Work out the finished part from the listing and answer in its coordinate system (mm). Coordinates: 2 decimals unless noted, no trailing zeros. Write each loop counter-clockwise with the first axis right and the second up, starting at its lowest first coordinate (ties: lowest second). Pieces come first, ordered by that corner, then holes. Notation, with made-up numbers: M 15,-26 L 54,-26 A11 cw 54,-12 Z; hole C -27.5,48 d2. An arc over 180 degrees is marked long. Answer as CSV lines item,"result". Start each with the question number.
(1) The mould has two halves that part along Z. Classify faces 1 (the cylindrical face through (-13, 1, -7)), 2 (the flat face through (-1, 0, -3)), 3 (the flat face through (36, 1, 29)): released by +Z, released by -Z, zero draft, split by the parting line, or undercut.
(2) A cutting plane is placed at A-A on x = -15. Give the vertices of the cut face in (y, z).
(3) A cutting plane is placed at D-D on y = 1.45. Count the separate pieces of the cut face and the enclosed holes in it, then the cut area to 3 significant figures.
(4) Find the intervals of material crossed by L1, parallel to Z at x = 10, y = 0.1; L2, parallel to Z at x = 14, y = 0.75; L3, parallel to Z at x = 47, y = 0.85, in increasing order. Write a range as [from, to].
(5) A cutting plane is placed at C-C on z = 25. Give the vertices of the cut face in (x, y), then the cut area to 3 significant figures.
(6) A cutting plane is placed at B-B on x = -46. Give the vertices of the cut face in (y, z).
(7) A flat-ended cylindrical pin translates along its axis: P1, Ø10, axis at x = 13.5, z = 6, coming from the -Y side. Find the tip coordinate at first contact, or state that the pin passes through.
from build123d import *

# Parameters (mm, degrees)
SKETCH_1_R      = 1.5
SKETCH_1_R_2    = 0.925
SKETCH_1_R_3    = 1
SKETCH_1_R_4    = 15
SKETCH_1_R_5    = 2.5
SKETCH_1_R_6    = 6.425
EXTRUDE_1_DEPTH = 2
FILLET_1_R      = 0.75


with BuildPart() as part:
    # 草图1 → 凸台-拉伸1 (new body)
    # profile 1 of 11: a face of its own
    with BuildSketch(Plane(origin=(0, 0, 0), x_dir=(1, 0, 0), z_dir=(0, 1, 0))):
        Polygon((-19.848034865, 26.695013128), (-30, 23), (30, 23), (19.848034865, 26.695013128), (0.026493373, 26.695013128), (-0.026493373, 26.695013128), align=None)
    # profile 2 of 11: a face of its own
    with BuildSketch(Plane(origin=(0, 0, 0), x_dir=(1, 0, 0), z_dir=(0, 1, 0))):
        Polygon((-19.848034865, 26.695013128), (-30, 23), (30, 23), (19.848034865, 26.695013128), (0.026493373, 26.695013128), (-0.026493373, 26.695013128), align=None)
    # profile 3 of 11: a face of its own
    with BuildSketch(Plane(origin=(0, 0, 0), x_dir=(1, 0, 0), z_dir=(0, 1, 0))):
        Polygon((-30, 23), (-50, 23), (-50, 7), (-50, -1), (-50, -5), (-50, -23), (-42, -23), (42, -23), (50, -23), (50, -5), (50, -1), (50, 7), (50, 23), (30, 23), align=None)
        with Locations(Location((-46, -15, 0), (0, 0, 270))):
            Circle(SKETCH_1_R, mode=Mode.SUBTRACT)
        with Locations(Location((-42, -15, 0), (0, 0, 270))):
            Circle(SKETCH_1_R_2, mode=Mode.SUBTRACT)
        with Locations(Location((-30.7465, -13.935, 0), (0, 0, 270))):
            Circle(SKETCH_1_R, mode=Mode.SUBTRACT)
        with Locations(Location((-12.727922061, -5.727922061, 0), (0, 0, 270))):
            Circle(SKETCH_1_R_3, mode=Mode.SUBTRACT)
        with BuildLine():
            ThreePointArc((-20.969611628, -19), (-22.969611628, -17), (-20.969611628, -15))
            Line((-20.969611628, -15), (20.969611628, -15))
            ThreePointArc((20.969611628, -15), (22.969611628, -17), (20.969611628, -19))
            Line((20.969611628, -19), (-20.969611628, -19))
        make_face(mode=Mode.SUBTRACT)
        with Locations(Location((30.7465, -13.935, 0), (0, 0, 270))):
            Circle(SKETCH_1_R, mode=Mode.SUBTRACT)
        with BuildLine():
            ThreePointArc((-6, -13), (-7.5, -11.5), (-6, -10))
            Line((-6, -10), (6, -10))
            ThreePointArc((6, -10), (7.5, -11.5), (6, -13))
            Line((6, -13), (-6, -13))
        make_face(mode=Mode.SUBTRACT)
        with Locations(Location((12.727922061, -5.727922061, 0), (0, 0, 270))):
            Circle(SKETCH_1_R_3, mode=Mode.SUBTRACT)
        with Locations(Location((42, -15, 0), (0, 0, 270))):
            Circle(SKETCH_1_R_2, mode=Mode.SUBTRACT)
        with Locations(Location((46, -15, 0), (0, 0, 270))):
            Circle(SKETCH_1_R, mode=Mode.SUBTRACT)
        with Locations(Location((-46, 0, 0), (0, 0, 270))):
            Circle(SKETCH_1_R, mode=Mode.SUBTRACT)
        with Locations(Location((-42, 0, 0), (0, 0, 270))):
            Circle(SKETCH_1_R_2, mode=Mode.SUBTRACT)
        with Locations(Location((-46, 15, 0), (0, 0, 270))):
            Circle(SKETCH_1_R, mode=Mode.SUBTRACT)
        with Locations(Location((-42, 15, 0), (0, 0, 270))):
            Circle(SKETCH_1_R_2, mode=Mode.SUBTRACT)
        with Locations(Location((-30.7465, 13.935, 0), (0, 0, 270))):
            Circle(SKETCH_1_R, mode=Mode.SUBTRACT)
        with Locations(Location((-12.727922061, 19.727922061, 0), (0, 0, 270))):
            Circle(SKETCH_1_R_3, mode=Mode.SUBTRACT)
        with Locations((0, 7)):
            Circle(SKETCH_1_R_4, mode=Mode.SUBTRACT)
        with Locations(Location((42, 0, 0), (0, 0, 270))):
            Circle(SKETCH_1_R_2, mode=Mode.SUBTRACT)
        with Locations(Location((46, 0, 0), (0, 0, 270))):
            Circle(SKETCH_1_R, mode=Mode.SUBTRACT)
        with Locations(Location((30.7465, 13.935, 0), (0, 0, 270))):
            Circle(SKETCH_1_R, mode=Mode.SUBTRACT)
        with Locations(Location((12.727922061, 19.727922061, 0), (0, 0, 270))):
            Circle(SKETCH_1_R_3, mode=Mode.SUBTRACT)
        with Locations(Location((42, 15, 0), (0, 0, 270))):
            Circle(SKETCH_1_R_2, mode=Mode.SUBTRACT)
        with Locations(Location((46, 15, 0), (0, 0, 270))):
            Circle(SKETCH_1_R, mode=Mode.SUBTRACT)
    # profile 4 of 11: a face of its own
    with BuildSketch(Plane(origin=(0, 0, 0), x_dir=(1, 0, 0), z_dir=(0, 1, 0))):
        Polygon((-30, 23), (-50, 23), (-50, 7), (-50, -1), (-50, -5), (-50, -23), (-42, -23), (42, -23), (50, -23), (50, -5), (50, -1), (50, 7), (50, 23), (30, 23), align=None)
        with Locations(Location((-46, -15, 0), (0, 0, 270))):
            Circle(SKETCH_1_R, mode=Mode.SUBTRACT)
        with Locations(Location((-42, -15, 0), (0, 0, 270))):
            Circle(SKETCH_1_R_2, mode=Mode.SUBTRACT)
        with Locations(Location((-30.7465, -13.935, 0), (0, 0, 270))):
            Circle(SKETCH_1_R, mode=Mode.SUBTRACT)
        with Locations(Location((-12.727922061, -5.727922061, 0), (0, 0, 270))):
            Circle(SKETCH_1_R_3, mode=Mode.SUBTRACT)
        with BuildLine():
            ThreePointArc((-20.969611628, -19), (-22.969611628, -17), (-20.969611628, -15))
            Line((-20.969611628, -15), (20.969611628, -15))
            ThreePointArc((20.969611628, -15), (22.969611628, -17), (20.969611628, -19))
            Line((20.969611628, -19), (-20.969611628, -19))
        make_face(mode=Mode.SUBTRACT)
        with Locations(Location((30.7465, -13.935, 0), (0, 0, 270))):
            Circle(SKETCH_1_R, mode=Mode.SUBTRACT)
        with BuildLine():
            ThreePointArc((-6, -13), (-7.5, -11.5), (-6, -10))
            Line((-6, -10), (6, -10))
            ThreePointArc((6, -10), (7.5, -11.5), (6, -13))
            Line((6, -13), (-6, -13))
        make_face(mode=Mode.SUBTRACT)
        with Locations(Location((12.727922061, -5.727922061, 0), (0, 0, 270))):
            Circle(SKETCH_1_R_3, mode=Mode.SUBTRACT)
        with Locations(Location((42, -15, 0), (0, 0, 270))):
            Circle(SKETCH_1_R_2, mode=Mode.SUBTRACT)
        with Locations(Location((46, -15, 0), (0, 0, 270))):
            Circle(SKETCH_1_R, mode=Mode.SUBTRACT)
        with Locations(Location((-46, 0, 0), (0, 0, 270))):
            Circle(SKETCH_1_R, mode=Mode.SUBTRACT)
        with Locations(Location((-42, 0, 0), (0, 0, 270))):
            Circle(SKETCH_1_R_2, mode=Mode.SUBTRACT)
        with Locations(Location((-46, 15, 0), (0, 0, 270))):
            Circle(SKETCH_1_R, mode=Mode.SUBTRACT)
        with Locations(Location((-42, 15, 0), (0, 0, 270))):
            Circle(SKETCH_1_R_2, mode=Mode.SUBTRACT)
        with Locations(Location((-30.7465, 13.935, 0), (0, 0, 270))):
            Circle(SKETCH_1_R, mode=Mode.SUBTRACT)
        with Locations(Location((-12.727922061, 19.727922061, 0), (0, 0, 270))):
            Circle(SKETCH_1_R_3, mode=Mode.SUBTRACT)
        with Locations((0, 7)):
            Circle(SKETCH_1_R_4, mode=Mode.SUBTRACT)
        with Locations(Location((42, 0, 0), (0, 0, 270))):
            Circle(SKETCH_1_R_2, mode=Mode.SUBTRACT)
        with Locations(Location((46, 0, 0), (0, 0, 270))):
            Circle(SKETCH_1_R, mode=Mode.SUBTRACT)
        with Locations(Location((30.7465, 13.935, 0), (0, 0, 270))):
            Circle(SKETCH_1_R, mode=Mode.SUBTRACT)
        with Locations(Location((12.727922061, 19.727922061, 0), (0, 0, 270))):
            Circle(SKETCH_1_R_3, mode=Mode.SUBTRACT)
        with Locations(Location((42, 15, 0), (0, 0, 270))):
            Circle(SKETCH_1_R_2, mode=Mode.SUBTRACT)
        with Locations(Location((46, 15, 0), (0, 0, 270))):
            Circle(SKETCH_1_R, mode=Mode.SUBTRACT)
    # profile 5 of 11: a face of its own
    with BuildSketch(Plane(origin=(0, 0, 0), x_dir=(1, 0, 0), z_dir=(0, 1, 0))):
        with Locations((0, 7)):
            Circle(SKETCH_1_R_4)
        with BuildLine():
            ThreePointArc((13, 7), (12.434860091, 3.208660592), (10.788576229, -0.253042323))
            ThreePointArc((10.788576229, -0.253042323), (9.192388155, -2.192388155), (7.253042323, -3.788576229))
            ThreePointArc((7.253042323, -3.788576229), (0, -6), (-7.253042323, -3.788576229))
            ThreePointArc((-7.253042323, -3.788576229), (-9.192388155, -2.192388155), (-10.788576229, -0.253042323))
            ThreePointArc((-10.788576229, -0.253042323), (-13, 7), (-10.788576229, 14.253042323))
            ThreePointArc((-10.788576229, 14.253042323), (-9.192388155, 16.192388155), (-7.253042323, 17.788576229))
            ThreePointArc((-7.253042323, 17.788576229), (0, 20), (7.253042323, 17.788576229))
            ThreePointArc((7.253042323, 17.788576229), (9.192388155, 16.192388155), (10.788576229, 14.253042323))
            ThreePointArc((10.788576229, 14.253042323), (12.434860091, 10.791339408), (13, 7))
        make_face(mode=Mode.SUBTRACT)
    # profile 6 of 11: a face of its own
    with BuildSketch(Plane(origin=(0, 0, 0), x_dir=(1, 0, 0), z_dir=(0, 1, 0))):
        with BuildLine():
            ThreePointArc((7.253042323, -3.788576229), (9.192388155, -2.192388155), (10.788576229, -0.253042323))
            Line((10.788576229, -0.253042323), (4.242640687, 6.292893219))
            ThreePointArc((4.242640687, 6.292893219), (3.949747468, 7), (4.242640687, 7.707106781))
            Line((4.242640687, 7.707106781), (10.788576229, 14.253042323))
            ThreePointArc((10.788576229, 14.253042323), (9.192388155, 16.192388155), (7.253042323, 17.788576229))
            Line((7.253042323, 17.788576229), (0.707106781, 11.242640687))
            ThreePointArc((0.707106781, 11.242640687), (0, 10.949747468), (-0.707106781, 11.242640687))
            Line((-0.707106781, 11.242640687), (-7.253042323, 17.788576229))
            ThreePointArc((-7.253042323, 17.788576229), (-9.192388155, 16.192388155), (-10.788576229, 14.253042323))
            Line((-10.788576229, 14.253042323), (-4.242640687, 7.707106781))
            ThreePointArc((-4.242640687, 7.707106781), (-3.949747468, 7), (-4.242640687, 6.292893219))
            Line((-4.242640687, 6.292893219), (-10.788576229, -0.253042323))
            ThreePointArc((-10.788576229, -0.253042323), (-9.192388155, -2.192388155), (-7.253042323, -3.788576229))
            Line((-7.253042323, -3.788576229), (-0.707106781, 2.757359313))
            ThreePointArc((-0.707106781, 2.757359313), (0, 3.050252532), (0.707106781, 2.757359313))
            Line((0.707106781, 2.757359313), (7.253042323, -3.788576229))
        make_face()
        with Locations(Location((-3.181980515, 3.818019485, 0), (0, 0, 270))):
            Circle(SKETCH_1_R_3, mode=Mode.SUBTRACT)
        with Locations(Location((-3.181980515, 10.181980515, 0), (0, 0, 270))):
            Circle(SKETCH_1_R_3, mode=Mode.SUBTRACT)
        with Locations(Location((3.181980515, 3.818019485, 0), (0, 0, 270))):
            Circle(SKETCH_1_R_3, mode=Mode.SUBTRACT)
        with Locations(Location((0, 7, 0), (0, 0, 270))):
            Circle(SKETCH_1_R_5, mode=Mode.SUBTRACT)
        with Locations(Location((3.181980515, 10.181980515, 0), (0, 0, 270))):
            Circle(SKETCH_1_R_3, mode=Mode.SUBTRACT)
    # profile 7 of 11: a face of its own
    with BuildSketch(Plane(origin=(0, 0, 0), x_dir=(1, 0, 0), z_dir=(0, 1, 0))):
        Polygon((42, -23), (-42, -23), (-30, -35), (30, -35), align=None)
        with BuildLine():
            ThreePointArc((-20.969611628, -31), (-22.969611628, -29), (-20.969611628, -27))
            Line((-20.969611628, -27), (20.969611628, -27))
            ThreePointArc((20.969611628, -27), (22.969611628, -29), (20.969611628, -31))
            Line((20.969611628, -31), (-20.969611628, -31))
        make_face(mode=Mode.SUBTRACT)
    # profile 8 of 11: a face of its own
    with BuildSketch(Plane(origin=(0, 0, 0), x_dir=(1, 0, 0), z_dir=(0, 1, 0))):
        Polygon((-50, -5), (-50, -1), (-58, 7), (-62, 7), align=None)
    # profile 9 of 11: a face of its own
    with BuildSketch(Plane(origin=(0, 0, 0), x_dir=(1, 0, 0), z_dir=(0, 1, 0))):
        Polygon((-50, 7), (-50, 23), (-66, 23), (-66, 7), (-62, 7), (-58, 7), align=None)
        with Locations(Location((-58, 15, 0), (0, 0, 270))):
            Circle(SKETCH_1_R_6, mode=Mode.SUBTRACT)
    # profile 10 of 11: a face of its own
    with BuildSketch(Plane(origin=(0, 0, 0), x_dir=(1, 0, 0), z_dir=(0, 1, 0))):
        Polygon((66, 23), (50, 23), (50, 7), (58, 7), (62, 7), (66, 7), align=None)
        with Locations(Location((58, 15, 0), (0, 0, 270))):
            Circle(SKETCH_1_R_6, mode=Mode.SUBTRACT)
    # profile 11 of 11: a face of its own
    with BuildSketch(Plane(origin=(0, 0, 0), x_dir=(1, 0, 0), z_dir=(0, 1, 0))):
        Polygon((58, 7), (50, -1), (50, -5), (62, 7), align=None)
    extrude(amount=EXTRUDE_1_DEPTH)

    # 圆角1
    fillet_1_edges = [part.edges().sort_by_distance(p)[0] for p in [
        (66, 1, -23),
        (66, 1, -7),
        (62, 1, -7),
        (50, 1, 5),
        (50, 1, 23),
        (42, 1, 23),
        (30, 1, 35),
        (-30, 1, 35),
        (-42, 1, 23),
        (-50, 1, 23),
        (-50, 1, 5),
        (-62, 1, -7),
        (-66, 1, -7),
        (50, 1, -7),
        (50, 1, 1),
        (58, 1, -7),
        (-50, 1, 1),
        (-50, 1, -7),
        (-58, 1, -7),
    ]]
    fillet(fillet_1_edges, radius=FILLET_1_R)


solid = part.part
Here are the results:
1,face 1,"undercut"
1,face 2,"zero draft"
1,face 3,"released by +Z"
2,outline,"M 0,-26.7 L 2,-26.7 L 2,15 L 0,15 Z; M 0,19 L 2,19 L 2,27 L 0,27 Z; M 0,31 L 2,31 L 2,35 L 0,35 Z"
3,separate pieces,"1"
3,enclosed holes,"36"
3,area,"5,150 mm^2"
4,L1,"z = [-26.7, -13.46], [-0.54, 15], [19, 27], [31, 35]"
4,L2,"z = [-26.7, 15], [19, 27], [31, 35]"
4,L3,"z = [-23, -16.12], [-13.88, -1.12], [1.12, 13.88], [16.12, 23]"
5,outline,"M -40,0 L 40,0 L 40,2 L -40,2 Z"
5,area,"160 mm^2"
6,outline,"M 0,-23 L 2,-23 L 2,-16.5 L 0,-16.5 Z; M 0,-13.5 L 2,-13.5 L 2,-1.5 L 0,-1.5 Z; M 0,1.5 L 2,1.5 L 2,13.5 L 0,13.5 Z; M 0,16.5 L 2,16.5 L 2,23 L 0,23 Z"
7,P1,"stops at y = 0"
